```python
from build123d import *

# Parameters (mm, degrees)
CROQUIS1_R              = 6.67
SALIENTE_EXTRUIR1_DEPTH = 62
CROQUIS2_R              = 4.61
SALIENTE_EXTRUIR2_DEPTH = 7.6
CROQUIS3_R              = 5.13
CORTAR_EXTRUIR1_DEPTH   = 60.6
CROQUIS4_R              = 3.07
CORTAR_EXTRUIR2_DEPTH   = 60.6
SALIENTE_EXTRUIR3_START = 1.54
CROQUIS5_W              = 13.34
CROQUIS5_H              = 27
CROQUIS5_R              = 5.13
SALIENTE_EXTRUIR3_DEPTH = 1.54
REDONDEO1_R             = 8


with BuildPart() as part:
    # Croquis1 → Saliente-Extruir1 (new body)
    with BuildSketch(Plane(origin=(0, 0, 0), x_dir=(1, 0, 0), z_dir=(0, 1, 0))):
        with Locations(Location((0, 0, 0), (0, 0, 270))):
            Circle(CROQUIS1_R)
    extrude(amount=SALIENTE_EXTRUIR1_DEPTH)

    # Croquis2 → Saliente-Extruir2 (add)
    with BuildSketch(Plane(origin=(0, 62, 0), x_dir=(1, 0, 0), z_dir=(0, 1, 0))):
        with Locations(Location((0, 0, 0), (0, 0, 90))):
            Circle(CROQUIS2_R)
    extrude(amount=SALIENTE_EXTRUIR2_DEPTH)

    # Croquis3 → Cortar-Extruir1 (cut)
    with BuildSketch(Plane.XZ):
        with Locations(Location((0, 0, 0), (0, 0, 270))):
            Circle(CROQUIS3_R)
    extrude(amount=-CORTAR_EXTRUIR1_DEPTH, mode=Mode.SUBTRACT)

    # Croquis4 → Cortar-Extruir2 (cut)
    with BuildSketch(Plane(origin=(0, 69.6, 0), x_dir=(1, 0, 0), z_dir=(0, 1, 0))):
        with Locations(Location((0, 0, 0), (0, 0, 270))):
            Circle(CROQUIS4_R)
    extrude(amount=-CORTAR_EXTRUIR2_DEPTH, mode=Mode.SUBTRACT)

    # Croquis5 → Saliente-Extruir3 (add)
    with BuildSketch(Plane.XZ.offset(SALIENTE_EXTRUIR3_START)):
        Rectangle(CROQUIS5_W, CROQUIS5_H)
        with Locations(Location((0, 0, 0), (0, 0, 270))):
            Circle(CROQUIS5_R, mode=Mode.SUBTRACT)
    extrude(amount=-SALIENTE_EXTRUIR3_DEPTH)

    # Redondeo1
    # the kernel refuses this fillet: 8 mm, written as the material it takes off along each edge
    with BuildSketch(Plane(origin=(-6.67, -21.54, -13.5), x_dir=(0, 0, 1), z_dir=(0, 1, 0)), Plane(origin=(6.67, -21.54, -13.5), x_dir=(-1, 0, 0), z_dir=(0, 1, 0)), Plane(origin=(6.67, -21.54, 13.5), x_dir=(0, 0, -1), z_dir=(0, 1, 0))) as redondeo1_piece_1:
        with BuildLine():
            CenterArc((REDONDEO1_R, REDONDEO1_R), REDONDEO1_R, 180, 90)
            Line((0, REDONDEO1_R), (0, 0))
            Line((0, 0), (REDONDEO1_R, 0))
        make_face()
    extrude(amount=41.54, mode=Mode.SUBTRACT)
    with BuildSketch(Plane(origin=(-6.67, -21.54, 13.5), x_dir=(0, 0, -1), z_dir=(0, 1, 0))) as redondeo1_piece_2:
        with BuildLine():
            CenterArc((REDONDEO1_R, -REDONDEO1_R), REDONDEO1_R, 90, 90)
            Line((0, -REDONDEO1_R), (0, 0))
            Line((0, 0), (REDONDEO1_R, 0))
        make_face()
    extrude(amount=41.54, mode=Mode.SUBTRACT)


solid = part.part
```
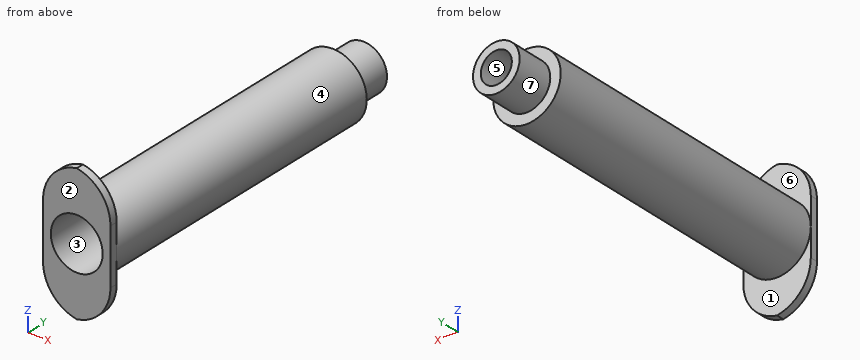
CAD build for the part. Positions are in the model's coordinates, mm. Face numbers are marked on the shaded views. A direction names the side the tool comes from. Coordinates: 2 decimals unless noted, no trailing zeros. Loops run counter-clockwise (first coordinate to the right, second up) from the corner with the lowest first, then second, coordinate; pieces in that order, holes last. Notation, with made-up numbers: (-1, 71.25) - (11, 71.25) arc R27 cw to (11, 103.25) - close; hole circle Ø2 at (-14.5, -5). An arc over 180 degrees is marked (long way). Use CSV: the item, a comma, the result in double quotes. Start each with the question number.
Q1. Drop flat-ended pins along their axis: P1, Ø10, axis at y = 16.5, z = 7, coming from the -X side; P2, Ø12, axis at y = 58, z = 6.5, coming from the -X side; P3, Ø5, axis at y = 59.5, z = 5.5, coming from the -X side; P4, Ø5, axis at x = 0, z = 0, coming from the -Y side. Give the stop position or say it passes through.
Q2. Two-plate mould, pull along Z, no slides. Class the marked faces 5, 6 and 7: +Z half, -Z half, draft (parallel to the pull), parting line (faces both ways), or undercut.
Q3. 3-axis set-ups, long thin cutter, end or side, ignore diameter. For the marked faces 1, 2, 3 and 4: which of +Z, -Z, +X, -X, +Y, -Y reach the whole face in a straight line?
Q4. Cut at D-D, the plane z = 9.75. List the corners of the cut face in (x, y).
Q5. Cut at B-B, the plane z = 0.75. List the corners of the cut face in (x, y), then the cut area to 3 significant figures.
Q6. Cut at A-A, the plane x = 2. List the corners of the cut face in (y, z).
Q7. Cut at C-C, the plane y = 20.5. List the corners of the cut face in (x, z), then the cut area to 3 significant figures.
Q8. Probe probe 1 along X at (y, z) = (17, 0); probe 2 along Y at (x, z) = (3.25, -11.5); probe 3 along Z at (x, y) = (0.25, 54). List the from-to ranges inside material, lowest first. Write a range as from..to.
Here are the results:
1,P1,"x = -6.36"
1,P2,"x = -6.65"
1,P3,"x = -5.96"
1,P4,"through"
2,face 5,"undercut"
2,face 6,"draft"
2,face 7,"parting line"
3,face 1,"-Z, +Y"
3,face 2,"+Z, -Z, +X, -X, -Y"
3,face 3,"-Y"
3,face 4,"+Y"
4,outline,"(-5.45, -1.54) - (5.45, -1.54) - (5.45, 0) - (-5.45, 0) - close"
5,outline,"(-6.67, -1.54) - (-5.07, -1.54) - (-5.07, 60.6) - (-2.98, 60.6) - (-2.98, 69.6) - (-4.55, 69.6) - (-4.55, 62) - (-6.63, 62) - (-6.63, 0) - (-6.67, 0) - close; (2.98, 60.6) - (5.07, 60.6) - (5.07, -1.54) - (6.67, -1.54) - (6.67, 0) - (6.63, 0) - (6.63, 62) - (4.55, 62) - (4.55, 69.6) - (2.98, 69.6) - close"
5,area,"227 mm2"
6,outline,"(-1.54, -12.77) - (0, -12.77) - (0, -6.36) - (62, -6.36) - (62, -4.15) - (69.6, -4.15) - (69.6, -2.33) - (60.6, -2.33) - (60.6, -4.72) - (-1.54, -4.72) - close; (-1.54, 4.72) - (60.6, 4.72) - (60.6, 2.33) - (69.6, 2.33) - (69.6, 4.15) - (62, 4.15) - (62, 6.36) - (0, 6.36) - (0, 12.77) - (-1.54, 12.77) - close"
7,outline,"circle Ø13.34 at (0, 0); hole circle Ø10.26 at (0, 0)"
7,area,"57.1 mm2"
8,probe 1,"-6.67..-5.13, 5.13..6.67"
8,probe 2,"-1.54..0"
8,probe 3,"-6.67..-5.12, 5.12..6.67"
